```python
from build123d import *

# Parameters (mm, degrees)
SCHIZZO1_W                   = 78
SCHIZZO1_H                   = 38
SCHIZZO1_R                   = 2.25
ESTRUSIONE_ESTRUSIONE1_DEPTH = 2
SCHIZZO2_W                   = 78
SCHIZZO2_H                   = 38
SCHIZZO2_R                   = 1.25
ESTRUSIONE_ESTRUSIONE2_DEPTH = 7
SCHIZZO3_W                   = 78
SCHIZZO3_H                   = 38
SCHIZZO3_W_2                 = 72
SCHIZZO3_H_2                 = 32
ESTRUSIONE_ESTRUSIONE3_DEPTH = 3
SMUSSO1_SIZE                 = 0.5
RACCORDO1_R                  = 5
SCHIZZO4_R                   = 4.5
TAGLIO_ESTRUSIONE1_DEPTH     = 1.5
RACCORDO2_R                  = 5
RACCORDO3_R                  = 1
TAGLIO_ESTRUSIONE2_REACH     = 57.758
SCHIZZO5_W                   = 7
SCHIZZO5_H                   = 7
RACCORDO4_R                  = 2.8
RACCORDO5_R                  = 0.2
RACCORDO6_R                  = 2


with BuildPart() as part:
    # Schizzo1 → Estrusione-Estrusione1 (new body)
    with BuildSketch(Plane.XY):
        Rectangle(SCHIZZO1_W, SCHIZZO1_H)
        with BuildLine():
            ThreePointArc((-34, 12.75), (-34.883883476, 14.883883476), (-32.75, 14))
            Line((-32.75, 14), (-34, 14))
            Line((-34, 14), (-34, 12.75))
        make_face(mode=Mode.SUBTRACT)
        with BuildLine():
            ThreePointArc((32.75, 14), (34.883883476, 14.883883476), (34, 12.75))
            Line((34, 12.75), (34, 14))
            Line((34, 14), (32.75, 14))
        make_face(mode=Mode.SUBTRACT)
        with BuildLine():
            ThreePointArc((34, -12.75), (34.883883476, -14.883883476), (32.75, -14))
            Line((32.75, -14), (34, -14))
            Line((34, -14), (34, -12.75))
        make_face(mode=Mode.SUBTRACT)
        with BuildLine():
            ThreePointArc((-32.75, -14), (-34.883883476, -14.883883476), (-34, -12.75))
            Line((-34, -12.75), (-34, -14))
            Line((-34, -14), (-32.75, -14))
        make_face(mode=Mode.SUBTRACT)
        with Locations((20, 10)):
            Circle(SCHIZZO1_R, mode=Mode.SUBTRACT)
        with Locations((-20, 10)):
            Circle(SCHIZZO1_R, mode=Mode.SUBTRACT)
        with Locations((20, -10)):
            Circle(SCHIZZO1_R, mode=Mode.SUBTRACT)
        with Locations((-20, -10)):
            Circle(SCHIZZO1_R, mode=Mode.SUBTRACT)
    extrude(amount=ESTRUSIONE_ESTRUSIONE1_DEPTH)

    # Schizzo2 → Estrusione-Estrusione2 (add)
    with BuildSketch(Plane.XY.offset(2)):
        Rectangle(SCHIZZO2_W, SCHIZZO2_H)
        with BuildLine():
            ThreePointArc((-36, 10.535898385), (-31.171572875, 11.171572875), (-30.535898385, 16))
            Line((-30.535898385, 16), (30.535898385, 16))
            ThreePointArc((30.535898385, 16), (31.171572875, 11.171572875), (36, 10.535898385))
            Line((36, 10.535898385), (36, -10.535898385))
            ThreePointArc((36, -10.535898385), (31.171572875, -11.171572875), (30.535898385, -16))
            Line((30.535898385, -16), (-30.535898385, -16))
            ThreePointArc((-30.535898385, -16), (-31.171572875, -11.171572875), (-36, -10.535898385))
            Line((-36, -10.535898385), (-36, 10.535898385))
        make_face(mode=Mode.SUBTRACT)
        with Locations((-34, 14)):
            Circle(SCHIZZO2_R, mode=Mode.SUBTRACT)
        with Locations((-34, -14)):
            Circle(SCHIZZO2_R, mode=Mode.SUBTRACT)
        with Locations(Location((34, -14, 0), (0, 0, 180))):
            Circle(SCHIZZO2_R, mode=Mode.SUBTRACT)
        with Locations(Location((34, 14, 0), (0, 0, 180))):
            Circle(SCHIZZO2_R, mode=Mode.SUBTRACT)
    extrude(amount=ESTRUSIONE_ESTRUSIONE2_DEPTH)

    # Schizzo3 → Estrusione-Estrusione3 (add)
    with BuildSketch(Plane.XY.offset(9)):
        Rectangle(SCHIZZO3_W, SCHIZZO3_H)
        Rectangle(SCHIZZO3_W_2, SCHIZZO3_H_2, mode=Mode.SUBTRACT)
    extrude(amount=ESTRUSIONE_ESTRUSIONE3_DEPTH)

    # Smusso1
    smusso1_edges = [part.edges().sort_by_distance(p)[0] for p in [
        (35.25, -14, 9),
        (-35.25, -14, 9),
        (-35.25, 14, 9),
        (35.25, 14, 9),
    ]]
    chamfer(smusso1_edges, length=SMUSSO1_SIZE)

    # Raccordo1
    raccordo1_edges = [part.edges().sort_by_distance(p)[0] for p in [
        (39, 19, 6),
        (39, -19, 6),
        (-39, -19, 6),
        (-39, 19, 6),
    ]]
    fillet(raccordo1_edges, radius=RACCORDO1_R)

    # Schizzo4 → Taglio-Estrusione1 (cut)
    with BuildSketch(Plane.XY.offset(2)):
        with Locations((-20, 10)):
            Circle(SCHIZZO4_R)
        with Locations((20, 10)):
            Circle(SCHIZZO4_R)
        with Locations((20, -10)):
            Circle(SCHIZZO4_R)
        with Locations((-20, -10)):
            Circle(SCHIZZO4_R)
    extrude(amount=-TAGLIO_ESTRUSIONE1_DEPTH, mode=Mode.SUBTRACT)

    # Raccordo2
    raccordo2_edges = [part.edges().sort_by_distance(p)[0] for p in [
        (30.535898385, 16, 5.5),
        (36, 10.535898385, 5.5),
        (36, -10.535898385, 5.5),
        (30.535898385, -16, 5.5),
        (-30.535898385, -16, 5.5),
        (-36, -10.535898385, 5.5),
        (-36, 10.535898385, 5.5),
        (-30.535898385, 16, 5.5),
    ]]
    fillet(raccordo2_edges, radius=RACCORDO2_R)

    # Raccordo3
    raccordo3_edges = [part.edges().sort_by_distance(p)[0] for p in [
        (-36, 16, 10.5),
        (-36, -16, 10.5),
        (36, -16, 10.5),
        (36, 16, 10.5),
    ]]
    fillet(raccordo3_edges, radius=RACCORDO3_R)

    # Schizzo5 → Taglio-Estrusione2 (cut, up to next)
    with BuildSketch(Plane(origin=(0, 19, 0), x_dir=(1, 0, 0), z_dir=(0, 1, 0)), mode=Mode.PRIVATE) as taglio_estrusione2_sk1:
        with Locations((0, -8.5)):
            Rectangle(SCHIZZO5_W, SCHIZZO5_H)
    taglio_estrusione2_tool1 = extrude(taglio_estrusione2_sk1.sketch, amount=-TAGLIO_ESTRUSIONE2_REACH, mode=Mode.PRIVATE) & part.part
    add(taglio_estrusione2_tool1.solids().sort_by_distance((0, 19, 8.5))[0], mode=Mode.SUBTRACT)

    # Raccordo4
    raccordo4_edges = [part.edges().sort_by_distance(p)[0] for p in [
        (3.5, 16, 8.5),
        (-3.5, 16, 8.5),
    ]]
    fillet(raccordo4_edges, radius=RACCORDO4_R)

    # Raccordo5
    raccordo5_edges = [part.edges().sort_by_distance(p)[0] for p in [
        (-3.5, 19, 8.5),
        (3.5, 19, 8.5),
    ]]
    fillet(raccordo5_edges, radius=RACCORDO5_R - 0.0001)  # a hair under: the kernel refuses the full size

    # Raccordo6
    raccordo6_edges = [part.edges().sort_by_distance(p)[0] for p in [
        (0, 16, 5),
    ]]
    fillet(raccordo6_edges, radius=RACCORDO6_R)


solid = part.part
```
The listing builds one solid part. Answer for the finished solid, in the listing's coordinates (mm). A direction names the side the tool comes from. Round coordinates to 2 decimals unless told otherwise and drop trailing zeros. Loops run counter-clockwise (first coordinate to the right, second up) from the corner with the lowest first, then second, coordinate; pieces in that order, holes last.
Q1. Section A-A, the plane x = 20 is taken. Determine the outline of the cut face in (y, z).
Q2. Find the intervals of material crossed by line 1 (Y direction, x = 20, z = 1); line 2 (X direction, y = 10, z = 11.5); line 3 (Y direction, x = 34, z = 3.5), in increasing order.
Q3. Section C-C, the plane z = 7.25 is taken. Count the separate pieces of the cut face and the enclosed holes in it, then the cut area to 3 significant figures.
Q4. Given pin 1 Ø5 at (x, y) = (28.5, 9.5) entering from +Z; pin 2 Ø1 at (x, y) = (33, -13.5) entering from +Z, each flat-ended and moving along its own axis, determine where each tip first touches the part or whether it passes through.
Q5. Which of the six approach directions +Z, -Z, +X, -X, +Y, -Y give full straight-line access (tool end or side, diameter ignored) to faces 1 (the face through (28.366, -15.107, 5.549)), 2 (the face through (-18.79, -8.103, 0.246))?
Q6. Section B-B, the plane y = -4.5 is taken. Determine the outline of the cut face in (x, z).
Q7. Section D-D, the plane y = 9 is taken. Determine the outline of the cut face in (x, z).
Q8. For a pull along Y with two mould halves and no side action, classify faces 3 (the face through (39, 0, 6)), 4 (the face through (-4.34, 16.8, 8.56)), 5 (the face through (0, -19, 6)) as released by +Y, released by -Y, zero draft, split by the parting line, or undercut.
Completed:
1. outline: (-19, 0) - (-12.25, 0) - (-12.25, 0.5) - (-14.5, 0.5) - (-14.5, 2) - (-16, 2) - (-16, 12) - (-19, 12) - close; (-7.75, 0) - (7.75, 0) - (7.75, 0.5) - (5.5, 0.5) - (5.5, 2) - (-5.5, 2) - (-5.5, 0.5) - (-7.75, 0.5) - close; (12.25, 0) - (19, 0) - (19, 12) - (16, 12) - (16, 2) - (14.5, 2) - (14.5, 0.5) - (12.25, 0.5) - close
2. line 1: y = -19 to -14.5, -5.5 to 5.5, 14.5 to 19
2. line 2: x = -39 to -36, 36 to 39
2. line 3: y = -19 to -15.25, -12.75 to -9.51, 9.51 to 12.75, 15.25 to 19
3. separate pieces: 1
3. enclosed holes: 4
3. area: 754 mm2
4. pin 1: stops at z = 2
4. pin 2: stops at z = 8.87
5. face 1: +Z
5. face 2: +Z, -Z
6. outline: (-39, 0) - (39, 0) - (39, 12) - (36, 12) - (36, 2) - (-36, 2) - (-36, 12) - (-39, 12) - close
7. outline: (-39, 0) - (-22.02, 0) - (-22.02, 0.5) - (-24.39, 0.5) - (-24.39, 2) - (-34.59, 2) - (-34.59, 9) - (-36, 9) - (-36, 12) - (-39, 12) - close; (-17.98, 0) - (17.98, 0) - (17.98, 0.5) - (15.61, 0.5) - (15.61, 2) - (-15.61, 2) - (-15.61, 0.5) - (-17.98, 0.5) - close; (22.02, 0) - (39, 0) - (39, 12) - (36, 12) - (36, 9) - (34.59, 9) - (34.59, 2) - (24.39, 2) - (24.39, 0.5) - (22.02, 0.5) - close
8. face 3: zero draft
8. face 4: undercut
8. face 5: released by -Y
